```python
from build123d import *

# Parameters (mm, degrees)
CROQUIS1_W              = 112
CROQUIS1_H              = 47
SALIENTE_EXTRUIR1_DEPTH = 87
CROQUIS2_R              = 10
CORTAR_EXTRUIR1_DEPTH   = 87
CORTAR_EXTRUIR2_DEPTH   = 87
CHAFL_N1_SIZE           = 0.4
CHAFL_N2_SIZE           = 0.4
REDONDEO1_R             = 1
REDONDEO2_R             = 1
SALIENTE_EXTRUIR2_DEPTH = 7
CROQUIS6_R              = 3.472712807
SALIENTE_EXTRUIR3_DEPTH = 1
CROQUIS7_R              = 5.694419986
SALIENTE_EXTRUIR4_DEPTH = 1
CROQUIS8_R              = 3.033642273
CROQUIS8_R_2            = 3.0923226
CORTAR_EXTRUIR3_DEPTH   = 3


with BuildPart() as part:
    # Croquis1 → Saliente-Extruir1 (new body)
    with BuildSketch(Plane.XY):
        Rectangle(CROQUIS1_W, CROQUIS1_H)
    extrude(amount=-SALIENTE_EXTRUIR1_DEPTH)

    # Croquis2 → Cortar-Extruir1 (cut)
    with BuildSketch(Plane.XY):
        with Locations((-39.5, 0)):
            Circle(CROQUIS2_R)
        with Locations(Location((39.5, 0, 0), (0, 0, 180))):
            Circle(CROQUIS2_R)
    extrude(amount=-CORTAR_EXTRUIR1_DEPTH, mode=Mode.SUBTRACT)

    # Croquis4 → Cortar-Extruir2 (cut)
    with BuildSketch(Plane(origin=(0, 0, -87), x_dir=(-1, 0, 0), z_dir=(0, 0, -1))):
        Polygon((10, 22.5), (-10, 22.5), (-10, 21.5), (-11, 21.5), (-11, 23.5), (0, 25.805357454), (11, 23.5), (11, 21.5), (10, 21.5), align=None)
    extrude(amount=-CORTAR_EXTRUIR2_DEPTH, mode=Mode.SUBTRACT)

    # Chaflán1
    chafl_n1_edges = [part.edges().sort_by_distance(p)[0] for p in [
        (-11, 21.5, -43.5),
        (-10, 21.5, -43.5),
    ]]
    chamfer(chafl_n1_edges, length=CHAFL_N1_SIZE)

    # Chaflán2
    chafl_n2_edges = [part.edges().sort_by_distance(p)[0] for p in [
        (10, 21.5, -43.5),
        (11, 21.5, -43.5),
    ]]
    chamfer(chafl_n2_edges, length=CHAFL_N2_SIZE)

    # Redondeo1
    redondeo1_edges = [part.edges().sort_by_distance(p)[0] for p in [
        (-33.5, 23.5, 0),
        (-33.5, 23.5, -87),
        (33.5, 23.5, 0),
        (33.5, 23.5, -87),
        (-56, 23.5, -43.5),
        (56, 23.5, -43.5),
    ]]
    fillet(redondeo1_edges, radius=REDONDEO1_R)

    # Redondeo2
    # the kernel refuses this fillet: 1 mm, written as the material it takes off along each edge
    with BuildSketch(Plane(origin=(-11, 23.5, -88.5), x_dir=(0, -1, 0), z_dir=(0, 0, 1))) as redondeo2_piece_1:
        with BuildLine():
            CenterArc((REDONDEO2_R, -REDONDEO2_R), REDONDEO2_R, 90, 90)
            Line((0, -REDONDEO2_R), (0, 0))
            Line((0, 0), (REDONDEO2_R, 0))
        make_face()
    extrude(amount=90, mode=Mode.SUBTRACT)
    with BuildSketch(Plane(origin=(11, 23.5, -88.5), x_dir=(0, -1, 0), z_dir=(0, 0, 1))) as redondeo2_piece_2:
        with BuildLine():
            CenterArc((REDONDEO2_R, REDONDEO2_R), REDONDEO2_R, 180, 90)
            Line((0, REDONDEO2_R), (0, 0))
            Line((0, 0), (REDONDEO2_R, 0))
        make_face()
    extrude(amount=90, mode=Mode.SUBTRACT)

    # Croquis5 → Saliente-Extruir2 (add)
    with BuildSketch(Plane(origin=(0, 23.5, 0), x_dir=(1, 0, 0), z_dir=(0, 1, 0))):
        Polygon((32.814266538, 66.19625833), (29.638840058, 71.69625833), (23.287987096, 71.69625833), (20.112560616, 66.19625833), (23.287987096, 60.69625833), (29.638840058, 60.69625833), align=None)
        Polygon((29.638840058, 26.30374167), (32.814266538, 20.80374167), (29.638840058, 15.30374167), (23.287987096, 15.30374167), (20.112560616, 20.80374167), (23.287987096, 26.30374167), align=None)
    extrude(amount=SALIENTE_EXTRUIR2_DEPTH)

    # Croquis6 → Saliente-Extruir3 (add)
    with BuildSketch(Plane(origin=(0, 30.5, 0), x_dir=(1, 0, 0), z_dir=(0, 1, 0))):
        with Locations(Location((26.463413577, 66.19625833, 0), (0, 0, 270))):
            Circle(CROQUIS6_R)
        with Locations(Location((26.463413577, 20.80374167, 0), (0, 0, 90))):
            Circle(CROQUIS6_R)
    extrude(amount=SALIENTE_EXTRUIR3_DEPTH)

    # Croquis7 → Saliente-Extruir4 (add)
    with BuildSketch(Plane(origin=(0, 31.5, 0), x_dir=(1, 0, 0), z_dir=(0, 1, 0))):
        with Locations(Location((26.463413577, 20.80374167, 0), (0, 0, 270))):
            Circle(CROQUIS7_R)
        with Locations(Location((26.463413577, 66.19625833, 0), (0, 0, 90))):
            Circle(CROQUIS7_R)
    extrude(amount=SALIENTE_EXTRUIR4_DEPTH)

    # Croquis8 → Cortar-Extruir3 (cut)
    with BuildSketch(Plane(origin=(0, 32.5, 0), x_dir=(1, 0, 0), z_dir=(0, 1, 0))):
        with Locations(Location((26.463413577, 20.80374167, 0), (0, 0, 270))):
            Circle(CROQUIS8_R)
        with Locations(Location((26.463413577, 66.19625833, 0), (0, 0, 270))):
            Circle(CROQUIS8_R_2)
    extrude(amount=-CORTAR_EXTRUIR3_DEPTH, mode=Mode.SUBTRACT)


solid = part.part
```
Input: part model. Units: mm. Frame: model coordinates. A direction names the side the tool comes from. Round coordinates to 2 decimals unless told otherwise and drop trailing zeros. Loops run counter-clockwise (first coordinate to the right, second up) from the corner with the lowest first, then second, coordinate; pieces in that order, holes last. Notation, with made-up numbers: (17, -11) -> (64, -11) arc R23 cw to (64, 16) -> close; hole circle Ø3 at (35.5, -13.75). An arc over 180 degrees is marked (long way). Use one line per item in the form item = value. Start each with the question number.
Item 1: Section query B-B on z = -76. Return the cut outline in (x, y).
Item 2: Section query D-D on x = -14.5. Return the cut outline in (y, z), then the cut area to 3 significant figures.
Item 3: Set-up query: faces 4 (the face through (21.72, 26.95, -18.02)), 5 (the face through (27, 29.5, -21)), 6 (the face through (26, 27, -60.696)). Return all of +Z, -Z, +X, -X, +Y, -Y with unobstructed straight access to the full face (end or side cutting, diameter ignored); none if empty.
Item 4: Mould query, pull axis Z, two halves, no side actions, for faces 1 (the face through (29, 31.5, -18)), 2 (the face through (49.49, -0.44, -42.89)), 3 (the face through (31.249, 26.951, -18.092)). Classes: pulls with the +Z half, pulls with the -Z half, needs draft (parallel to the pull), parting line crosses it, or undercut.
Item 5: Section query C-C on x = -39.5. Return the cut outline in (y, z), then the cut area to 3 significant figures.
Item 6: Contact query for flat-ended pins moving along their axis: pin 1 Ø5 at (x, y) = (28, 27.5) entering from -Z; pin 2 Ø10 at (x, z) = (1.5, -32) entering from +Y; pin 3 Ø12 at (x, z) = (25, -64.5) entering from +Y; pin 4 Ø7 at (x, y) = (25.5, 27.5) entering from +Z. Output: stop coordinate, or through.
Item 7: Material intervals for L1, parallel to Y at x = -39.5, z = -56.5; L2, parallel to X at y = 8, z = -64; L3, parallel to Y at x = 0.5, z = -72, sorted ascending. Write a range as from..to.
Item 8: Section query A-A on y = 0. Return the cut outline in (x, z), then the cut area to 3 significant figures.
Ans:
q1.outline = (-56, -23.5) -> (56, -23.5) -> (56, 22.5) arc R1 ccw to (55, 23.5) -> (12, 23.5) arc R1 ccw to (11, 22.5) -> (11, 21.9) -> (10.6, 21.5) -> (10.4, 21.5) -> (10, 21.9) -> (10, 22.5) -> (-10, 22.5) -> (-10, 21.9) -> (-10.4, 21.5) -> (-10.6, 21.5) -> (-11, 21.9) -> (-11, 22.5) arc R1 ccw to (-12, 23.5) -> (-55, 23.5) arc R1 ccw to (-56, 22.5) -> close; hole circle Ø20 at (-39.5, 0); hole circle Ø20 at (39.5, 0)
q2.outline = (-23.5, -87) -> (22.5, -87) arc R1 ccw to (23.5, -86) -> (23.5, -1) arc R1 ccw to (22.5, 0) -> (-23.5, 0) -> close
q2.area = 4,090 mm^2
q3.face_4 = +Z, -X
q3.face_5 = +Y
q3.face_6 = +X, -X
q4.face_1 = undercut
q4.face_2 = needs draft
q4.face_3 = pulls with the +Z half
q5.outline = (-23.5, -87) -> (-10, -87) -> (-10, 0) -> (-23.5, 0) -> close; (10, -87) -> (22.5, -87) arc R1 ccw to (23.5, -86) -> (23.5, -1) arc R1 ccw to (22.5, 0) -> (10, 0) -> close
q5.area = 2,350 mm^2
q6.pin_1 = -71.7
q6.pin_2 = 22.5
q6.pin_3 = 32.5
q6.pin_4 = -15.3
q7.L1 = -23.5..-10, 10..23.5
q7.L2 = -56..-45.5, -33.5..33.5, 45.5..56
q7.L3 = -23.5..22.5
q8.outline = (-56, -87) -> (-49.5, -87) -> (-49.5, 0) -> (-56, 0) -> close; (-29.5, -87) -> (29.5, -87) -> (29.5, 0) -> (-29.5, 0) -> close; (49.5, -87) -> (56, -87) -> (56, 0) -> (49.5, 0) -> close
q8.area = 6,260 mm^2
